```python
from build123d import *

# Parameters (mm, degrees)
SKETCH1_W              = 152.4
SKETCH1_H              = 209.55
BOSS_EXTRUDE2_DEPTH    = 5.08
SKETCH2_R              = 8.73125
CUT_EXTRUDE1_DEPTH     = 6.08
F_10_CLEARANCE_HOLE2_D = 5.1054
FILLET1_R              = 4.445
F_10_CLEARANCE_HOLE1_D = 5.1054


with BuildPart() as part:
    # Sketch1 → Boss-Extrude2 (new body)
    with BuildSketch(Plane(origin=(0, 0, 0), x_dir=(0, 0, -1), z_dir=(1, 0, 0))):
        with Locations((76.2, 104.775)):
            Rectangle(SKETCH1_W, SKETCH1_H)
    extrude(amount=BOSS_EXTRUDE2_DEPTH)

    # Sketch2 → Cut-Extrude1 (cut, through all)
    with BuildSketch(Plane(origin=(5.08, 0, 0), x_dir=(0, 0, -1), z_dir=(1, 0, 0))):
        with Locations((76.2, 50.8)):
            Circle(SKETCH2_R)
    extrude(amount=-CUT_EXTRUDE1_DEPTH, mode=Mode.SUBTRACT)

    # #10 Clearance Hole2 (through all)
    with Locations(Plane(origin=(5.08, 0, 0), x_dir=(0, 0, -1), z_dir=(1, 0, 0))):
        with Locations((48.520375625, 68.0466), (74.555375625, 144.106959494), (100.590375625, 82.55), (74.555375625, 28.575)):
            Hole(F_10_CLEARANCE_HOLE2_D / 2)

    # Fillet1
    fillet1_edges = [part.edges().sort_by_distance(p)[0] for p in [
        (2.54, 209.55, 0),
        (2.54, 209.55, -152.4),
        (2.54, 0, -152.4),
        (2.54, 0, 0),
    ]]
    fillet(fillet1_edges, radius=FILLET1_R)

    # #10 Clearance Hole1 (through all)
    with Locations(Plane(origin=(5.08, 0, 0), x_dir=(0, 0, -1), z_dir=(1, 0, 0))):
        with Locations((6.35, 203.2), (146.05, 6.35), (6.35, 6.35), (146.05, 203.2), (76.2, 6.35), (76.2, 203.2), (6.35, 137.583333333), (6.35, 71.966666667), (146.05, 71.966666667), (146.05, 137.583333333)):
            Hole(F_10_CLEARANCE_HOLE1_D / 2)


solid = part.part
```
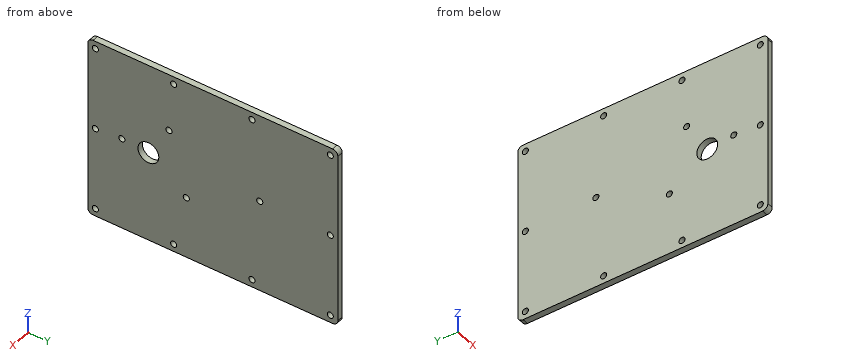
Geometry check sheet. Reference: the model listing, model coordinates, mm. Coordinates: 2 decimals unless noted, no trailing zeros. Loops run counter-clockwise (first coordinate to the right, second up) from the corner with the lowest first, then second, coordinate; pieces in that order, holes last. Notation, with made-up numbers: (-28, 0.5) -> (-14, 0.5) arc R20 ccw to (-14, 14.5) -> close; hole circle Ø5 at (-31.5, -27.75). An arc over 180 degrees is marked (long way). Put each result on its own line as item: value.
1) Cross-section at B-B on x = 1.2. Count the separate pieces of the cut face and the enclosed holes in it, plus the area to 3 significant figures.
Result set:
separate pieces: 1
enclosed holes: 15
area: 31,400 mm^2
2) Gauge pin test, flat end, axial feed: pin 1 Ø6.5 at (y, z) = (6.35, -76.2) entering from -X. Record the tip position at first contact, or that the pin passes through.
Result set:
pin 1: stops at x = 0
3) Cross-section at A-A on y = 50.8. Record the boundary of the cut face in (x, z), plus the area to 3 significant figures.
Result set:
outline: (0, -152.4) -> (5.08, -152.4) -> (5.08, -84.93) -> (0, -84.93) -> close; (0, -67.47) -> (5.08, -67.47) -> (5.08, 0) -> (0, 0) -> close
area: 685 mm^2
4) Thickness scan on line 1 (Z direction, x = 2.3, y = 203.2); line 2 (Z direction, x = 3.95, y = 139.5); line 3 (Z direction, x = 3.6, y = 26.5). Record the ranges inside material, lowest first.
Result set:
line 1: z = -152.4 to -148.6, -143.5 to -78.75, -73.65 to -8.9, -3.8 to 0
line 2: z = -152.4 to -147.74, -144.36 to -8.04, -4.66 to 0
line 3: z = -152.4 to -76.04, -73.07 to 0
